from build123d import *

# Parameters (mm, degrees)
SKETCH_R            = 2.5
PAD_DEPTH           = 1.5
SKETCH001_R         = 2.65
HOLE_DEPTH          = 25
LINEARPATTERN_COUNT = 7
LINEARPATTERN_PITCH = 116.666667


with BuildPart() as part:
    # Sketch → Pad (new body)
    with BuildSketch(Plane.XY):
        with BuildLine():
            Line((0, -3), (0, -80))
            Line((-37, -80), (0, -80))
            ThreePointArc((-45, -72), (-42.656854, -77.656854), (-37, -80))
            Line((-45, -72), (-45, 41))
            ThreePointArc((-37, 49), (-42.656854, 46.656854), (-45, 41))
            Line((-37, 49), (877, 49))
            ThreePointArc((885, 41), (882.656854, 46.656854), (877, 49))
            Line((885, 41), (885, -72))
            ThreePointArc((877, -80), (882.656854, -77.656854), (885, -72))
            Line((877, -80), (800, -80))
            Line((800, -80), (800, -3))
            ThreePointArc((800, -3), (799.12132, -0.87868), (797, 0))
            Line((797, 0), (3, 0))
            ThreePointArc((3, 0), (0.87868, -0.87868), (0, -3))
        make_face()
        with Locations((-37, 41)):
            Circle(SKETCH_R, mode=Mode.SUBTRACT)
        with Locations((-37, -72)):
            Circle(SKETCH_R, mode=Mode.SUBTRACT)
        with Locations((877, -72)):
            Circle(SKETCH_R, mode=Mode.SUBTRACT)
        with Locations((877, 41)):
            Circle(SKETCH_R, mode=Mode.SUBTRACT)
    extrude(amount=PAD_DEPTH)

    # Sketch001 → Hole (cut)
    with BuildSketch(Plane.XY.offset(2)):
        with Locations((50, 12.5)):
            Circle(SKETCH001_R)
    hole = extrude(amount=-HOLE_DEPTH, mode=Mode.SUBTRACT)

    # LinearPattern: Hole ×7
    with Locations(*[(i * LINEARPATTERN_PITCH, 0, 0) for i in range(1, LINEARPATTERN_COUNT)]):
        add(hole, mode=Mode.SUBTRACT)


solid = part.part
Input: part model. Units: mm. Frame: model coordinates. Round coordinates to 2 decimals unless told otherwise and drop trailing zeros. Order: outer loops, then holes, each group sorted by start corner. A loop starts at its lowest first (then second) coordinate and runs counter-clockwise, first axis right, second up. Notation, with made-up numbers: (62, -13) - (103, -13) arc R8 cw to (103, -2) - close; hole circle Ø11 at (81.5, 69). An arc over 180 degrees is marked (long way). Answer as a JSON object with one key per item and string values. Group by question number.
(1) Cut plane A-A (y = -41). Return loops of the section in (x, z), then the cut area to 3 significant figures.
(2) Pin query (flat end, axial travel): P1, Ø0.8, axis at x = 367.5, z = 1, coming from the -Y side. Return the tip coordinate at first contact, or that it passes through.
(3) Cut plane B-B (z = 1.2). Count the separate pieces of the cut face and the enclosed holes in it, then the cut area to 3 significant figures.
(4) Material intervals for probe 1 along Y at (x, z) = (-37, 1.15); probe 2 along X at (y, z) = (-63, 0.75); probe 3 along Y at (x, z) = (441, 0.1), sorted ascending. Write a range as from..to.
(5) Cut plane C-C (x = 104). Return loops of the section in (y, z).
Here are the results:
{
 "1": {"outline": "(-45, 0) - (0, 0) - (0, 1.5) - (-45, 1.5) - close; (800, 0) - (885, 0) - (885, 1.5) - (800, 1.5) - close", "area": "195 mm^2"},
 "2": {"P1": "stops at y = 0"},
 "3": {"separate pieces": "1", "enclosed holes": "11", "area": "55,700 mm^2"},
 "4": {"probe 1": "y = -80..-74.5, -69.5..38.5, 43.5..49", "probe 2": "x = -45..0, 800..885", "probe 3": "y = 0..49"},
 "5": {"outline": "(0, 0) - (49, 0) - (49, 1.5) - (0, 1.5) - close"}
}
